```python
from build123d import *

# Parameters (mm, degrees)
SKETCH_1_R          = 250
EXTRUDE_2_DEPTH     = 30
FILLET_1_R          = 30
SKETCH_4_R          = 80
EXTRUDE_4_DEPTH     = 300
SKETCH_5_R          = 12
EXTRUDE_6_DEPTH     = 45
SKETCH_6_R          = 10
CUT_EXTRUDE_2_DEPTH = 45


with BuildPart() as part:
    # 草图1 → 凸台-拉伸2 (new body)
    with BuildSketch(Plane(origin=(0, 0, 0), x_dir=(1, 0, 0), z_dir=(0, 1, 0))):
        with Locations(Location((0, 0, 0), (0, 0, 270))):
            Circle(SKETCH_1_R)
    extrude(amount=EXTRUDE_2_DEPTH)

    # 圆角1
    fillet_1_edges = [part.edges().sort_by_distance(p)[0] for p in [
        (0, 30, -250),
    ]]
    fillet(fillet_1_edges, radius=FILLET_1_R - 0.0001)  # a hair under: the kernel refuses the full size

    # 草图4 → 凸台-拉伸4 (add)
    with BuildSketch(Plane(origin=(0, 30, 0), x_dir=(1, 0, 0), z_dir=(0, 1, 0))):
        with Locations(Location((0, 0, 0), (0, 0, 270))):
            Circle(SKETCH_4_R)
    extrude(amount=EXTRUDE_4_DEPTH)

    # 草图5 → 凸台-拉伸6 (add)
    with BuildSketch(Plane(origin=(0, 330, 0), x_dir=(1, 0, 0), z_dir=(0, 1, 0))):
        with Locations(Location((0, 0, 0), (0, 0, 90))):
            Circle(SKETCH_5_R)
    extrude(amount=EXTRUDE_6_DEPTH)

    # 草图6 → 切除-拉伸2 (cut)
    with BuildSketch(Plane(origin=(0, 375, 0), x_dir=(1, 0, 0), z_dir=(0, 1, 0))):
        with Locations(Location((0, 0, 0), (0, 0, 270))):
            Circle(SKETCH_6_R)
    extrude(amount=-CUT_EXTRUDE_2_DEPTH, mode=Mode.SUBTRACT)


solid = part.part
```
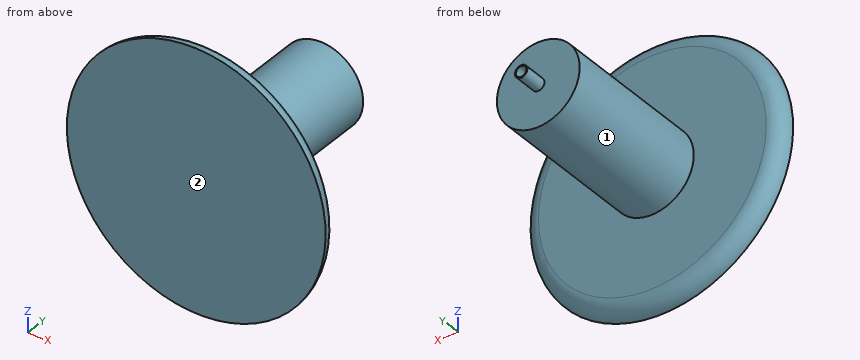
The model under review builds one solid part; all positions refer to its coordinate system, in mm. Face numbers are marked on the shaded views. A direction names the side the tool comes from. Round coordinates to 2 decimals unless told otherwise and drop trailing zeros. Order: outer loops, then holes, each group sorted by start corner. A loop starts at its lowest first (then second) coordinate and runs counter-clockwise, first axis right, second up. Notation, with made-up numbers: (-2, -15.75) -> (33, -15.75) arc R19 ccw to (33, 18.25) -> close; hole circle Ø1 at (67.25, 43.5). An arc over 180 degrees is marked (long way). One line per item, written item: value. Start each with the question number.
Q1. Clearance check with flat-ended pins moving along their axes: pin 1 Ø1 at (x, z) = (10.5, -181) entering from +Y; pin 2 Ø6 at (x, z) = (0, -0.5) entering from +Y; pin 3 Ø10 at (y, z) = (143, 74.5) entering from +X; pin 4 Ø1 at (x, z) = (-100.5, 151) entering from -Y. State where each tip first meets the part, or that it passes through.
Q2. Machinability: for the marked faces 1 and 2, which of the approach directions +Z, -Z, +X, -X, +Y, -Y give a long, thin tool a straight path to every point of the face, cutting with its end or side? Answer none if there is none.
Q3. Wall thickness on line 1 (X direction, y = 357, z = 0); line 2 (Y direction, x = -91, z = 18.5); line 3 (Y direction, x = 11, z = -62.5): over which ranges is each line inside the solid? List them lowest first.
Q4. Take a section at B-B (y = 44.5). Write out the cut boundary in (x, z).
Reported:
1. pin 1: stops at y = 30
1. pin 2: stops at y = 330
1. pin 3: stops at x = 39.62
1. pin 4: stops at y = 0
2. face 1: +Y
2. face 2: +Z, -Z, +X, -X, -Y
3. line 1: x = -12 to -10, 10 to 12
3. line 2: y = 0 to 30
3. line 3: y = 0 to 330
4. outline: circle Ø160 at (0, 0)
